```python
from build123d import *

# Parameters (mm, degrees)
SKETCH2_W           = 10
SKETCH2_H           = 50
BOSS_EXTRUDE1_DEPTH = 10
SKETCH6_R           = 2.35
CUT_EXTRUDE3_DEPTH  = 11
SKETCH7_R           = 2.35
CUT_EXTRUDE4_DEPTH  = 11
SKETCH8_W           = 1.5
SKETCH8_H           = 21
BOSS_EXTRUDE2_DEPTH = 30
SKETCH9_W           = 52.99414334
SKETCH9_H           = 19.059793282
CUT_EXTRUDE5_DEPTH  = 11


with BuildPart() as part:
    # Sketch2 → Boss-Extrude1 (new body)
    with BuildSketch(Plane.XY):
        with Locations((5, 25)):
            Rectangle(SKETCH2_W, SKETCH2_H)
    extrude(amount=BOSS_EXTRUDE1_DEPTH)

    # Sketch6 → Cut-Extrude3 (cut, through all)
    with BuildSketch(Plane.XY.offset(10)):
        with Locations((5, 27)):
            Circle(SKETCH6_R)
    extrude(amount=-CUT_EXTRUDE3_DEPTH, mode=Mode.SUBTRACT)

    # Sketch7 → Cut-Extrude4 (cut, through all)
    with BuildSketch(Plane.ZY):
        with Locations((5, 41)):
            Circle(SKETCH7_R)
        with Locations((5, 9)):
            Circle(SKETCH7_R)
    extrude(amount=-CUT_EXTRUDE4_DEPTH, mode=Mode.SUBTRACT)

    # Sketch8 → Boss-Extrude2 (add)
    with BuildSketch(Plane.ZY):
        with Locations((9.25, 26)):
            Rectangle(SKETCH8_W, SKETCH8_H)
        with Locations((0.75, 26)):
            Rectangle(SKETCH8_W, SKETCH8_H)
    extrude(amount=BOSS_EXTRUDE2_DEPTH)

    # Sketch9 → Cut-Extrude5 (cut, through all)
    with BuildSketch(Plane.XY.offset(10)):
        with Locations((-7.642110933, 41.529896641)):
            Rectangle(SKETCH9_W, SKETCH9_H)
    extrude(amount=-CUT_EXTRUDE5_DEPTH, mode=Mode.SUBTRACT)


solid = part.part
```
Can you work these out from the model? Positions are in its coordinate system, mm. A direction names the side the tool comes from. Round coordinates to 2 decimals unless told otherwise and drop trailing zeros. Loops run counter-clockwise (first coordinate to the right, second up) from the corner with the lowest first, then second, coordinate; pieces in that order, holes last. Notation, with made-up numbers: (16.25, 32.25) -> (28.25, 32.25) arc R20 ccw to (28.25, 36.25) -> close; hole circle Ø5 at (53.5, -6.5). An arc over 180 degrees is marked (long way). One line per item, written item: value. Start each with the question number.
1. If we section it at D-D, the plane y = 9: Write out the boundary of the cut face in (x, z).
2. If I drill on probe 1 along Z at (x, y) = (-1, 22); probe 2 along Y at (x, z) = (5, 7.5); probe 3 along Y at (x, z) = (5, 3.75), over which ranges is the centre line in solid material (lowest first)?
3. For faces 4 (the cylindrical face through (6.084, 24.915, 5.07)), 5 (the flat face through (-15, 24, 8.5)), 6 (the flat face through (-15, 15.5, 1)), which set-ups out of +Z, -Z, +X, -X, +Y, -Y let a thin tool reach every point of the face, with its end or its side?
4. If we section it at A-A, the plane x = 5: Write out the boundary of the cut face in (y, z), then the cut area to 3 significant figures.
5. If we section it at C-C, the plane x = -2.5: Write out the boundary of the cut face in (y, z), then the cut area to 3 significant figures.
6. For pin 1 (18 mm diameter, centred on x = -14.5, y = 20, fed in from -Z); pin 2 (1.2 mm diameter, centred on x = -10.5, z = 9, fed in from -Y); pin 3 (3 mm diameter, centred on y = 9, z = 5, fed in from -X), each with a flat end and sliding along its axis, tell me the tip position at first contact or that it passes through.
7. If we mould it in two halves opening along Z, with no side actions, what happens to faces 1 (the cylindrical face through (4.93, 8.1, 7.17)), 2 (the flat face through (-30, 24, 1)), 3 (the flat face through (-10, 20, 0))? For each: pulls with the +Z half, pulls with the -Z half, needs draft (parallel to the pull), parting line crosses it, or undercut.
8. If we section it at B-B, the plane z = 5: Write out the boundary of the cut face in (x, y), then the cut area to 3 significant figures.
Calculated:
1. outline: (0, 0) -> (10, 0) -> (10, 2.65) -> (0, 2.65) -> close; (0, 7.35) -> (10, 7.35) -> (10, 10) -> (0, 10) -> close
2. probe 1: z = 0 to 1.5, 8.5 to 10
2. probe 2: y = 0 to 24.65, 29.35 to 32
2. probe 3: y = 0 to 7.01, 10.99 to 24.65, 29.35 to 32
3. face 4: +Z, -Z
3. face 5: -X, +Y, -Y
3. face 6: +Z, -Z, -X, -Y
4. outline: (0, 0) -> (24.65, 0) -> (24.65, 10) -> (0, 10) -> close; (29.35, 0) -> (32, 0) -> (32, 10) -> (29.35, 10) -> close; hole circle Ø4.7 at (9, 5)
4. area: 256 mm²
5. outline: (15.5, 0) -> (32, 0) -> (32, 1.5) -> (15.5, 1.5) -> close; (15.5, 8.5) -> (32, 8.5) -> (32, 10) -> (15.5, 10) -> close
5. area: 49.5 mm²
6. pin 1: stops at z = 0
6. pin 2: stops at y = 15.5
6. pin 3: passes through
7. face 1: undercut
7. face 2: needs draft
7. face 3: pulls with the -Z half
8. outline: (0, 0) -> (10, 0) -> (10, 6.65) -> (0, 6.65) -> close; (0, 11.35) -> (10, 11.35) -> (10, 32) -> (0, 32) -> close; hole circle Ø4.7 at (5, 27)
8. area: 256 mm²
